from build123d import *

# Parameters (mm, degrees)
BOSS_EXTRUDE1_DEPTH     = 30
SKETCH2_R               = 11
CUT_EXTRUDE1_DEPTH      = 8
SKETCH3_R               = 1.3
CUT_EXTRUDE2_DEPTH      = 1
CUT_EXTRUDE2_DEPTH_BACK = 175
SKETCH4_W               = 4
SKETCH4_H               = 10
CUT_EXTRUDE3_DEPTH      = 1
CUT_EXTRUDE3_DEPTH_BACK = 175
SKETCH5_R               = 21
CUT_EXTRUDE4_DEPTH      = 2


with BuildPart() as part:
    # Sketch1 → Boss-Extrude1 (new body)
    with BuildSketch(Plane.XY):
        Polygon((-87, 20), (-87, 0), (87, 0), (87, 20), (86, 20), (86, 10), (-86, 10), (-86, 20), align=None)
    extrude(amount=BOSS_EXTRUDE1_DEPTH)

    # Sketch2 → Cut-Extrude1 (cut)
    with BuildSketch(Plane(origin=(0, 10, 0), x_dir=(1, 0, 0), z_dir=(0, 1, 0))):
        with Locations((0, -15)):
            Circle(SKETCH2_R)
    extrude(amount=-CUT_EXTRUDE1_DEPTH, mode=Mode.SUBTRACT)

    # Sketch3 → Cut-Extrude2 (cut, two sides)
    with BuildSketch(Plane(origin=(87, 0, 0), x_dir=(0, 0, -1), z_dir=(1, 0, 0))) as cut_extrude2_sk:
        with Locations((-23, 15)):
            Circle(SKETCH3_R)
        with Locations((-7, 15)):
            Circle(SKETCH3_R)
    extrude(amount=CUT_EXTRUDE2_DEPTH, mode=Mode.SUBTRACT)
    extrude(cut_extrude2_sk.sketch, amount=-CUT_EXTRUDE2_DEPTH_BACK, mode=Mode.SUBTRACT)

    # Sketch4 → Cut-Extrude3 (cut, two sides)
    with BuildSketch(Plane.ZY.offset(87)) as cut_extrude3_sk:
        with Locations((15, 15)):
            Rectangle(SKETCH4_W, SKETCH4_H)
    extrude(amount=CUT_EXTRUDE3_DEPTH, mode=Mode.SUBTRACT)
    extrude(cut_extrude3_sk.sketch, amount=-CUT_EXTRUDE3_DEPTH_BACK, mode=Mode.SUBTRACT)

    # Sketch5 → Cut-Extrude4 (cut)
    with BuildSketch(Plane(origin=(0, 10, 0), x_dir=(1, 0, 0), z_dir=(0, 1, 0))):
        with Locations((0, -15)):
            Circle(SKETCH5_R)
    extrude(amount=-CUT_EXTRUDE4_DEPTH, mode=Mode.SUBTRACT)


solid = part.part
Read the model definition and answer for the solid it produces. Units are mm, in the model's axes. A direction names the side the tool comes from. Give positions to 0.01 mm unless a question says otherwise; leave off trailing zeros. Loops run counter-clockwise (first coordinate to the right, second up) from the corner with the lowest first, then second, coordinate; pieces in that order, holes last. Notation, with made-up numbers: (-16.75, 10.25) -> (34.25, 10.25) arc R18 cw to (34.25, 20.25) -> close; hole circle Ø4 at (48, 81.25). An arc over 180 degrees is marked (long way). Answer as CSV lines item,"result".
Item 1: Each of these flat-tipped pins is pushed along its axis until it touches: pin 1 (6.5 mm diameter, centred on x = 2, z = 11.5, fed in from +Y); pin 2 (10 mm diameter, centred on x = -58, z = 4, fed in from +Y). Where does it stop, or does it pass through?
Returned:
pin 1,"stops at y = 2"
pin 2,"stops at y = 10"
Item 2: Find section B-B on x = 0. Give the vertices of the cut face in (y, z), plus the area to 3 significant figures.
Returned:
outline,"(0, 0) -> (8, 0) -> (8, 4) -> (2, 4) -> (2, 26) -> (8, 26) -> (8, 30) -> (0, 30) -> close"
area,"108 mm²"
Item 3: For faces 4 (the face through (-1, 6, 30)), 5 (the face through (-86, 15, 5)), 6 (the face through (-2.38, 5.04, 25.74)), determine the directions among +Z, -Z, +X, -X, +Y, -Y from which every point of the face is accessible in a straight line to the end or side of a thin tool.
Returned:
face 4,"+Z, +X, -X, +Y, -Y"
face 5,"+Z, -Z, +Y"
face 6,"+Y"
Item 4: Consider line 1 (Y direction, x = 86.3, z = 7); line 2 (Z direction, x = 0, y = 6.8); line 3 (X direction, y = 15.5, z = 28). Determine where each line is inside the solid, lowest interval first. Write a range as [from, to].
Returned:
line 1,"y = [0, 13.7], [16.3, 20]"
line 2,"z = [0, 4], [26, 30]"
line 3,"x = [-87, -86], [86, 87]"
Item 5: Determine the mould class of faces 1 (the face through (50, 10, 15)), 2 (the face through (-1, 0, 15)), 3 (the face through (-87, 8, 15)) for opening direction X: +X half, -X half, draft (parallel to the pull), parting line (faces both ways), or undercut.
Returned:
face 1,"undercut"
face 2,"draft"
face 3,"-X half"
Item 6: Find section C-C on z = 15. Give the vertices of the cut face in (x, y), plus the area to 3 significant figures.
Returned:
outline,"(-87, 0) -> (87, 0) -> (87, 10) -> (21, 10) -> (21, 8) -> (11, 8) -> (11, 2) -> (-11, 2) -> (-11, 8) -> (-21, 8) -> (-21, 10) -> (-87, 10) -> close"
area,"1,520 mm²"
Item 7: Find section D-D on x = -72.5. Give the vertices of the cut face in (y, z), plus the area to 3 significant figures.
Returned:
outline,"(0, 0) -> (10, 0) -> (10, 30) -> (0, 30) -> close"
area,"300 mm²"
Item 8: Find section A-A on y = 17.75. Give the vertices of the cut face in (x, z), plus the area to 3 significant figures.
Returned:
outline,"(-87, 0) -> (-86, 0) -> (-86, 13) -> (-87, 13) -> close; (-87, 17) -> (-86, 17) -> (-86, 30) -> (-87, 30) -> close; (86, 0) -> (87, 0) -> (87, 13) -> (86, 13) -> close; (86, 17) -> (87, 17) -> (87, 30) -> (86, 30) -> close"
area,"52.0 mm²"
